from build123d import *

# Parameters (mm, degrees)
F1_DEPTH = 38.0422770977
F2_R     = 5.08
F3_DEPTH = 12.232337147
F4_R     = 5.08
F5_DEPTH = 7.3413159698
F6_DEPTH = 8.9663118124


with BuildPart() as f1:
    # F0 (on Top) → F1 (new body)
    with BuildSketch(Plane.XY):
        Polygon((43.8701745906, -1.9375651716), (14.2481029034, 14.3980756402), (-7.7989399433, -16.04783535), (19.3933885201, -35.7388352654), align=None)
    extrude(amount=F1_DEPTH)

    # F2
    f2_edges = [f1.edges().sort_by_distance(p)[0] for p in [
        (31.631782, -18.8382, 38.042277),
        (29.059139, 6.230255, 38.042277),
        (3.224581, -0.82488, 38.042277),
        (5.797224, -25.893335, 38.042277),
    ]]
    fillet(f2_edges, radius=F2_R)

    # F3 (add): a face of the model
    f3_faces = [f1.faces().sort_by_distance(p)[0] for p in [
        (17.578761895, -9.9497918988, 38.0422770977),
    ]]
    extrude(f3_faces, amount=F3_DEPTH)

    # F4
    f4_edges = [f1.edges().sort_by_distance(p)[0] for p in [
        (7.511612, -3.566101, 50.274614),
        (8.776694, -21.77883, 50.274614),
        (27.322154, -16.128185, 50.274614),
        (26.057072, 2.084544, 50.274614),
    ]]
    fillet(f4_edges, radius=F4_R)

    # F5 (add): a face of the model
    f5_faces = [f1.faces().sort_by_distance(p)[0] for p in [
        (17.4849129571, -9.9130484235, 50.2746142447),
    ]]
    extrude(f5_faces, amount=F5_DEPTH)

    # F6 (add): a face of the model
    f6_faces = [f1.faces().sort_by_distance(p)[0] for p in [
        (17.4849129571, -9.9130484235, 57.6159302145),
    ]]
    extrude(f6_faces, amount=F6_DEPTH)


solid = f1.part
Source: CAD feature listing. Evaluate the final solid. Frame: model axes, mm. A direction names the side the tool comes from. Give positions to 0.01 mm unless a question says otherwise; leave off trailing zeros. Write each loop counter-clockwise with the first axis right and the second up, starting at its lowest first coordinate (ties: lowest second). Pieces come first, ordered by that corner, then holes. Notation, with made-up numbers: M -5.75,-36.5 L 4.25,-36.5 A12 cw 4.25,-31.5 Z; hole C 10.5,35.5 d10. An arc over 180 degrees is marked long. Return JSON: item names as keys, results as strings. Group by question number.
1) Cut plane B-B, the plane z = 21.5. Output: boundary loops of the cut face in (x, y).
2) First-contact query: pin 1 Ø5 at (y, z) = (-2.5, 53) entering from -X; pin 2 Ø1.5 at (x, z) = (10.5, 7.5) entering from -Y; pin 3 Ø1 at (y, z) = (0, 21) entering from -X. Flat tips, straight axial feed; report the tip coordinate or a pass-through.
3) Ray query, L1, parallel to X at y = -20, z = 14.5; L2, parallel to Z at x = 30, y = -13.5; L3, parallel to Y at x = 32, z = 42.5. Return the intervals inside material, ascending.
4) Set-up query: faces 1 (the face through (23.14, -2.11, 58.31)), 2 (the face through (27.2, -16.3, 41.6)), 3 (the face through (8.64, -21.68, 41.57)), 4 (the face through (11.874, -6.203, 58.314)). Return all of +Z, -Z, +X, -X, +Y, -Y with unobstructed straight access to the full face (end or side cutting, diameter ignored); none if empty.
5) Cut plane A-A, the plane z = 61.5. Output: boundary loops of the cut face in (x, y).
Data:
{
 "1": {"outline": "M -7.8,-16.05 L 19.39,-35.74 L 43.87,-1.94 L 14.25,14.4 Z"},
 "2": {"pin 1": "stops at x = 12.75", "pin 2": "stops at y = -29.84", "pin 3": "stops at x = 3.46"},
 "3": {"L1": "x = -2.34 to 30.79", "L2": "z = 0 to 38", "L3": "y = -9.67 to -1.19"},
 "4": {"face 1": "+Z, +X, +Y", "face 2": "+Z, +X, -Y", "face 3": "+Z, -X, -Y", "face 4": "+Z, -X, +Y"},
 "5": {"outline": "M 6.39,-13.78 L 17.12,-21.55 L 28.9,-5.29 L 17.21,1.16 Z"}
}
